Autodesk Inventor part; units mm, degrees
ref_plane "作業平面1" through (0, 0, -6.7) normal (0, 0, -1) x (-1, 0, 0)
ref_plane "YZ Plane" through (0, 0, 0) normal (1, 0, 0) x (0, 1, 0)
ref_plane "XZ Plane" through (0, 0, 0) normal (0, 1, 0) x (-1, 0, 0)
sketch "スケッチ1" plane through (0, 0, 0) normal (0, 0, 1) x (1, 0, 0)
  line L0 (-19, 8.4016) -> (-19, -8.0875) construction
  line L1 (0, -8.2446) -> (0, 8.2446) construction
  line L2 (8.7, 8.4016) -> (8.7, -8.0875) construction
  circle A0 centre (0, 0) radius 6.05
  line L3 (6.05, 6.05) -> (-16.45, 6.05)
  line L4 (-16.45, 6.05) -> (-16.45, -6.05)
  line L5 (-16.45, -6.05) -> (6.05, -6.05)
  line L6 (6.05, -6.05) -> (6.05, 6.05)
  point P0 (6.05, 0)
  dimension "HEIGHT" = 12.1
  dimension "d0" = 8.7
  dimension "d1" = 27.7
  dimension "WIDTH" = 22.5
extrude "軸台" add sketch "スケッチ1" along normal blind 3 contours A0
extrude "本体" add sketch "スケッチ1" against normal blind 23.4
ref_plane "作業平面1" through (0, 0, -6.7) normal (0, 0, -1) x (-1, 0, 0)
sketch "スケッチ2" plane through (0, 0, -6.7) normal (0, 0, -1) x (-1, 0, 0)
  line L0 (-11, 6.05) -> (21.3, 6.05)
  line L1 (21.3, 6.05) -> (21.3, -6.05)
  line L2 (21.3, -6.05) -> (-11, -6.05)
  line L3 (-11, -6.05) -> (-11, 6.05)
  line L4 (-6.05, 6.05) -> (0, 6.05)
  line L5 (0, -6.05) -> (-6.05, -6.05)
  circle A0 centre (19, 0) radius 1.1
  circle A1 centre (-8.7, 0) radius 1.1
  line L6 (-8.7, 8.0806) -> (-8.7, -7.6301) construction
  line L7 (19, -7.6301) -> (19, 8.0806) construction
  line L8 (5.15, 8.0806) -> (5.15, -7.8882) construction
  line L9 (-11, 0.9) -> (-9.3325, 0.9)
  line L10 (-9.3325, 0.9) -> (-9.3325, -0.9)
  line L11 (-9.3325, -0.9) -> (-11, -0.9)
  line L12 (-11, -0.9) -> (-11, 0.9)
  line L13 (19.6325, 0.9) -> (21.3, 0.9)
  line L14 (21.3, 0.9) -> (21.3, -0.9)
  line L15 (21.3, -0.9) -> (19.6325, -0.9)
  line L16 (19.6325, -0.9) -> (19.6325, 0.9)
  point P0 (0, 0)
  point P1 (5.15, 6.05)
  point P2 (-11, 0)
  point P3 (21.3, 0)
  dimension "d10" = 2.2
  dimension "d9" = 32.3
  dimension "d11" = 8.7
  dimension "d12" = 27.7
  dimension "d13" = 1.8
extrude "タブ" add sketch "スケッチ2" against normal blind 2.5 contours L0 L1 L13 A0 L15 L2 L3 L11 A1 L9
sketch "スケッチ3" plane through (0, 0, 3) normal (0, 0, 1) x (1, 0, 0)
  circle A0 centre (0, 0) radius 2.43
  dimension "d16" = 4.86
extrude "軸" add sketch "スケッチ3" along normal blind 3
equation "\"d12\" = d1"
properties part number "FS90R"
Geometry: final body of the model. Coordinates: model frame, mm. A direction names the side the tool comes from. Round coordinates to 2 decimals unless told otherwise and drop trailing zeros. Order: outer loops, then holes, each group sorted by start corner. A loop starts at its lowest first (then second) coordinate and runs counter-clockwise, first axis right, second up. Notation, with made-up numbers: (7.5, -17.5) -> (12.5, -17.5) arc R20 cw to (12.5, -6.5) -> close; hole circle Ø7 at (20.25, 11.5). An arc over 180 degrees is marked (long way). Use CSV: the item, a comma, the result in double quotes. Start each with the question number.
1) Section A-A (x = 8.7). Return the cut outline in (y, z).
2) Set-up query: faces 4 (the face through (10, 0.9, -5)), 5 (the face through (5.589, 2.317, 1.479)), 6 (the face through (6.05, 0, -15)), 7 (the face through (-20, 0.9, -5)), 8 (the face through (6.05, 0, -2)). Return all of +Z, -Z, +X, -X, +Y, -Y with unobstructed straight access to the full face (end or side cutting, diameter ignored); none if empty.
3) Section C-C (z = -15.5). Return the cut outline in (x, y), and give its area (3 significant figures).
4) Draft query along Z for faces 1 (the face through (-18.8, 1.4, -4.2)), 2 (the face through (7, 0, -6.7)), 3 (the face through (-20, -0.9, -5)). Return one class per face: +Z half, -Z half, draft (parallel to the pull), parting line (faces both ways), or undercut.
5) First-contact query: pin 1 Ø3.5 at (x, y) = (-10.5, 3) entering from +Z; pin 2 Ø5.5 at (x, y) = (8.5, -0.5) entering from +Z; pin 3 Ø3.5 at (y, z) = (1, -15.5) entering from -X. Flat tips, straight axial feed; report the tip coordinate or a pass-through.
6) Material intervals for line 1 along Y through (x, z) = (8.7, -5.1); line 2 along Z through (x, y) = (3, -2.25); line 3 along Z through (x, y) = (-15, 1), sorted ascending. Write a range as from..to.
Returned:
1,outline,"(-6.05, -6.7) -> (-1.1, -6.7) -> (-1.1, -4.2) -> (-6.05, -4.2) -> close; (1.1, -6.7) -> (6.05, -6.7) -> (6.05, -4.2) -> (1.1, -4.2) -> close"
2,face 4,"+Z, -Z, +X"
2,face 5,"+Z"
2,face 6,"-Z, +X, +Y, -Y"
2,face 7,"+Z, -Z, -X"
2,face 8,"+Z, +X, +Y, -Y"
3,outline,"(-16.45, -6.05) -> (6.05, -6.05) -> (6.05, 6.05) -> (-16.45, 6.05) -> close"
3,area,"272 mm²"
4,face 1,"+Z half"
4,face 2,"-Z half"
4,face 3,"draft"
5,pin 1,"stops at z = 0"
5,pin 2,"stops at z = 3"
5,pin 3,"stops at x = -16.45"
6,line 1,"y = -6.05..-1.1, 1.1..6.05"
6,line 2,"z = -23.4..3"
6,line 3,"z = -23.4..0"
